Source: CAD feature listing. Evaluate the final solid. Frame: model axes, mm. Face numbers are marked on the shaded views. Give positions to 0.01 mm unless a question says otherwise; leave off trailing zeros. Write each loop counter-clockwise with the first axis right and the second up, starting at its lowest first coordinate (ties: lowest second). Pieces come first, ordered by that corner, then holes. Notation, with made-up numbers: M 19.25,62 L 28.25,62 A34 cw 28.25,101 Z; hole C 78,7 d11. An arc over 180 degrees is marked long. Use CSV: the item, a comma, the result in double quotes. Start each with the question number.
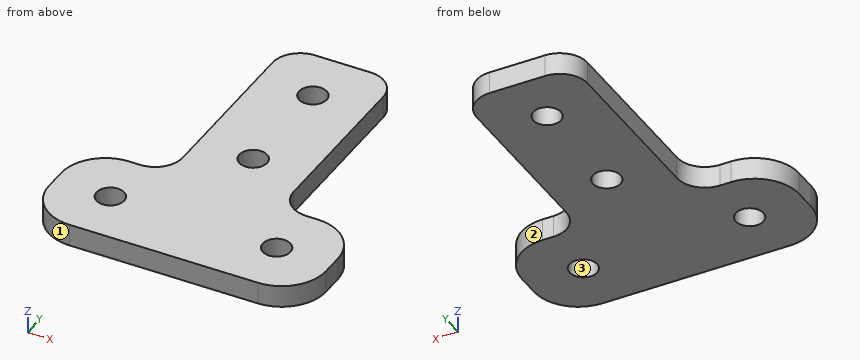
from build123d import *

# Parameters (mm, degrees)
SKETCH1_R           = 2.5
BOSS_EXTRUDE1_DEPTH = 4
FILLET1_R           = 5
FILLET2_R           = 8


with BuildPart() as part:
    # Sketch1 → Boss-Extrude1 (new body)
    with BuildSketch(Plane.XY):
        Polygon((-10, 60), (10, 60), (10, 20), (25, 20), (25, 0), (-25, 0), (-25, 20), (-10, 20), align=None)
        with Locations((0, 50)):
            Circle(SKETCH1_R, mode=Mode.SUBTRACT)
        with Locations((0, 30)):
            Circle(SKETCH1_R, mode=Mode.SUBTRACT)
        with Locations((15, 10)):
            Circle(SKETCH1_R, mode=Mode.SUBTRACT)
        with Locations((-15, 10)):
            Circle(SKETCH1_R, mode=Mode.SUBTRACT)
    extrude(amount=BOSS_EXTRUDE1_DEPTH)

    # Fillet1
    fillet1_edges = [part.edges().sort_by_distance(p)[0] for p in [
        (-10, 20, 2),
        (-10, 60, 2),
        (10, 60, 2),
        (10, 20, 2),
    ]]
    fillet(fillet1_edges, radius=FILLET1_R)

    # Fillet2
    fillet2_edges = [part.edges().sort_by_distance(p)[0] for p in [
        (25, 0, 2),
        (-25, 0, 2),
        (-25, 20, 2),
        (25, 20, 2),
    ]]
    fillet(fillet2_edges, radius=FILLET2_R)


solid = part.part
1. First-contact query: pin 1 (0.6 mm diameter, centred on x = -15.5, z = 3, fed in from +Y); pin 2 (2 mm diameter, centred on y = 41, z = 2, fed in from -X); pin 3 (4 mm diameter, centred on x = 0, y = 50, fed in from +Z); pin 4 (8 mm diameter, centred on x = -15, y = 10, fed in from +Z). Flat tips, straight axial feed; report the tip coordinate or a pass-through.
2. Section B-B on z = 0.8. Return loops of the section in (x, y).
3. Line query: probe 1 along Y at (x, z) = (0, 2.2); probe 2 along Y at (x, z) = (-15, 2.6); probe 3 along X at (y, z) = (54, 0.3). Output: solid intervals per line, ascending.
4. Section D-D on x = -18.5. Return loops of the section in (y, z).
5. Pull-direction query (X, two-part tool) for the marked faces 1, 2 and 3; classes: released by +X, released by -X, zero draft, split by the parting line, or undercut.
6. Section A-A on x = 0. Return loops of the section in (y, z).
7. Section C-C on y = 50. Return loops of the section in (x, z), then the cut area to 3 significant figures.
Resolved:
1,pin 1,"stops at y = 20"
1,pin 2,"stops at x = -10"
1,pin 3,"passes through"
1,pin 4,"stops at z = 4"
2,outline,"M -25,8 A8 ccw -17,0 L 17,0 A8 ccw 25,8 L 25,12 A8 ccw 17,20 L 15,20 A5 cw 10,25 L 10,55 A5 ccw 5,60 L -5,60 A5 ccw -10,55 L -10,25 A5 cw -15,20 L -17,20 A8 ccw -25,12 Z; hole C -15,10 d5; hole C 0,30 d5; hole C 0,50 d5; hole C 15,10 d5"
3,probe 1,"y = 0 to 27.5, 32.5 to 47.5, 52.5 to 60"
3,probe 2,"y = 0 to 7.5, 12.5 to 20"
3,probe 3,"x = -10 to 10"
4,outline,"M 0.14,0 L 19.86,0 L 19.86,4 L 0.14,4 Z"
5,face 1,"released by -X"
5,face 2,"released by +X"
5,face 3,"undercut"
6,outline,"M 0,0 L 27.5,0 L 27.5,4 L 0,4 Z; M 32.5,0 L 47.5,0 L 47.5,4 L 32.5,4 Z; M 52.5,0 L 60,0 L 60,4 L 52.5,4 Z"
7,outline,"M -10,0 L -2.5,0 L -2.5,4 L -10,4 Z; M 2.5,0 L 10,0 L 10,4 L 2.5,4 Z"
7,area,"60.0 mm2"
